Verification items for the finished model (mm, model axes). A direction names the side the tool comes from. Give positions to 0.01 mm unless a question says otherwise; leave off trailing zeros. Loops run counter-clockwise (first coordinate to the right, second up) from the corner with the lowest first, then second, coordinate; pieces in that order, holes last. Notation, with made-up numbers: (-17, -10) - (42, -10) arc R23 ccw to (42, 29) - close; hole circle Ø6 at (1, 76.5). An arc over 180 degrees is marked (long way). Answer in a Markdown table with one row per item.
```python
from build123d import *

# Parameters (mm, degrees)
F1_DEPTH  = 76.2
F2_R      = 23.0023216087
F3_DEPTH  = 63.501
F4_W      = 11.9801070541
F4_H      = 57.9038551077
F5_DEPTH  = 50.8
F6_W      = 33.9436382055
F6_H      = 64.7496273741
F7_DEPTH  = 17.78
F8_R      = 12.7
F9_DEPTH  = 76.2
F10_W     = 38.1
F10_H     = 25.4
F11_DEPTH = 63.5
F12_R     = 8.1391487304
F13_DEPTH = 50.8
F14_R     = 4.7187063419
F15_DEPTH = 50.8
F16_W     = 6.577372551
F16_H     = 31.1278868467
F17_DEPTH = 50.8
F19_DEPTH = 30.48
F20_W     = 76.2
F20_H     = 25.4
F21_DEPTH = 88.9


with BuildPart() as f1:
    # F0 (on Front) → F1 (new body)
    with BuildSketch(Plane.XZ):
        Polygon((-45.5546230793, -12.3941076807), (-45.5546230793, -37.7941076807), (43.3453769207, -37.7941076807), (43.3453769207, -12.3941076807), (17.9453769207, -12.3941076807), (17.9453769207, 51.1058923193), (43.3453769207, 51.1058923193), (43.3453769207, 76.5058923193), (-45.5546230793, 76.5058923193), (-45.5546230793, 51.1058923193), (-20.1546230793, 51.1058923193), (-20.1546230793, -12.3941076807), align=None)
    extrude(amount=F1_DEPTH)

    # F2 (on face) → F3 (cut, through all)
    with BuildSketch(Plane.YZ.offset(17.9453769207)):
        with Locations((-38.1, 19.3558923193)):
            Circle(F2_R)
    extrude(amount=-F3_DEPTH, mode=Mode.SUBTRACT)

    # F4 (on face) → F5 (join)
    with BuildSketch(Plane.XY.offset(76.5058923193)):
        with Locations((-26.5273796394, -38.7927298434)):
            Rectangle(F4_W, F4_H)
    extrude(amount=F5_DEPTH)

    # F6 (on face) → F7 (cut)
    with BuildSketch(Plane.XY.offset(76.5058923193)):
        with Locations((21.820910275, -37.3665248044)):
            Rectangle(F6_W, F6_H)
    extrude(amount=-F7_DEPTH, mode=Mode.SUBTRACT)

    # F8 (on face) → F9 (join)
    with BuildSketch(Plane.XY.offset(58.7258923193)):
        with Locations((22.248769179, -38.9353483915)):
            Circle(F8_R)
    extrude(amount=F9_DEPTH)

    # F10 (on face) → F11 (join)
    with BuildSketch(Plane(origin=(-32.5174331665, 0, 0), x_dir=(0, -1, 0), z_dir=(-1, 0, 0))):
        with Locations((46.303805925, 104.9945801497)):
            Rectangle(F10_W, F10_H)
    extrude(amount=F11_DEPTH)

    # F12 (on face) → F13 (join)
    with BuildSketch(Plane.XY.offset(134.9258923193)):
        with Locations((22.248769179, -38.9353483915)):
            Circle(F12_R)
    extrude(amount=F13_DEPTH)

    # F14 (on face) → F15 (join)
    with BuildSketch(Plane.XY.offset(185.7258923193)):
        with Locations((22.248769179, -38.9353483915)):
            Circle(F14_R)
    extrude(amount=F15_DEPTH)

    # F16 (on face) → F17 (join)
    with BuildSketch(Plane.XY.offset(127.3058923193)):
        with Locations((-23.8260123879, -42.9039588198)):
            Rectangle(F16_W, F16_H)
    extrude(amount=F17_DEPTH)

    # F18 (on face) → F19 (cut)
    with BuildSketch(Plane(origin=(-27.1146986634, 0, 0), x_dir=(0, -1, 0), z_dir=(-1, 0, 0))):
        Polygon((41.9095075075, 171.2333210797), (32.5746728326, 135.9694041327), (52.8574562847, 134.7401379139), align=None)
    extrude(amount=-F19_DEPTH, mode=Mode.SUBTRACT)

    # F20 (on face) → F21 (join)
    with BuildSketch(Plane.YZ.offset(43.3453769207)):
        with Locations((-38.1, -25.0941076807)):
            Rectangle(F20_W, F20_H)
    extrude(amount=F21_DEPTH)


solid = f1.part
```
Q1. Sectioned sample at B-B (x = 97.5). Record the cut outline in (y, z), and give its area (3 significant figures).
Completed:
| item | result |
|---|---|
| outline | (-76.2, -37.79) - (0, -37.79) - (0, -12.39) - (-76.2, -12.39) - close |
| area | 1,940 mm^2 |
Q2. Tool access check on faces 1 (the face through (38.793, -38, 68)), 2 (the face through (-64, -46, 92.295)), 3 (the face through (-64, -65.354, 105)), 4 (the face through (74, -39, -12.394)). Record the directions out of +Z, -Z, +X, -X, +Y, -Y that give a thin tool (end or side, any length) a straight path to the whole face; none if there is none.
Completed:
| item | result |
|---|---|
| face 1 | +Z |
| face 2 | -X, +Y, -Y |
| face 3 | +Z, -X, -Y |
| face 4 | +X, +Y, -Y |
Q3. Draft check along Y on faces 5 (the face through (-27, -67.745, 102)), 6 (the face through (-23.87, -47.46, 152.73)), 7 (the face through (43.345, -38, 64)). Enter one of: +Y half, -Y half, draft (parallel to the pull), parting line (faces both ways), or undercut.
Completed:
| item | result |
|---|---|
| face 5 | -Y half |
| face 6 | undercut |
| face 7 | draft |
Q4. Thickness scan on line 1 (Z direction, x = 18.5, y = -19.5); line 2 (Z direction, x = 0, y = -38.1); line 3 (X direction, y = -23.5, z = 69.5). Record the ranges inside material, lowest first.
Completed:
| item | result |
|---|---|
| line 1 | -37.79 to -12.39, 51.11 to 58.73 |
| line 2 | -37.79 to -3.65, 42.36 to 76.51 |
| line 3 | -45.55 to 4.85, 38.79 to 43.35 |
Q5. Go/stop test with flat-tipped pins: P1, Ø7, axis at x = -24, z = 146.5, coming from the +Y side; P2, Ø17.5, axis at y = -25, z = 148, coming from the +X side; P3, Ø8, axis at x = 45.5, y = -56.5, coming from the +Z side. Record where each tip stops, or that it passes through.
Completed:
| item | result |
|---|---|
| P1 | y = -27.34 |
| P2 | x = 28.52 |
| P3 | z = 76.51 |
Q6. Sectioned sample at A-A (z = 98.5). Record the cut outline in (x, y).
Completed:
| item | result |
|---|---|
| outline | (-96.02, -65.35) - (-32.52, -65.35) - (-32.52, -67.74) - (-20.54, -67.74) - (-20.54, -9.84) - (-32.52, -9.84) - (-32.52, -27.25) - (-96.02, -27.25) - close; circle Ø25.4 at (22.25, -38.94) |
